Read the model definition and answer for the solid it produces. Units are mm, in the model's axes. A direction names the side the tool comes from. Give positions to 0.01 mm unless a question says otherwise; leave off trailing zeros. Order: outer loops, then holes, each group sorted by start corner. A loop starts at its lowest first (then second) coordinate and runs counter-clockwise, first axis right, second up.
```python
from build123d import *

# Parameters (mm, degrees)
SKETCH2_W           = 98
SKETCH2_H           = 62
BOSS_EXTRUDE1_DEPTH = 25
SKETCH3_W           = 9.5
SKETCH3_H           = 12
BOSS_EXTRUDE4_DEPTH = 1
SKETCH3_5_W         = 9.5
SKETCH3_5_H         = 12
CUT_EXTRUDE1_DEPTH  = 1
SKETCH4_R           = 3.25
CUT_EXTRUDE2_DEPTH  = 10
SKETCH5_R           = 0.5
BOSS_EXTRUDE5_DEPTH = 8
SKETCH6_W           = 7
SKETCH6_H           = 14
CUT_EXTRUDE9_DEPTH  = 10
SKETCH7_W           = 1.559437484
SKETCH7_H           = 10
BOSS_EXTRUDE6_DEPTH = 9
SKETCH8_W           = 15
SKETCH8_H           = 10
BOSS_EXTRUDE7_DEPTH = 2
BOSS_EXTRUDE7_TAPER = 30
FILLET5_R           = 2
SKETCH10_R          = 2.5
CUT_EXTRUDE10_DEPTH = 6
SKETCH11_R          = 0.5
CUT_EXTRUDE11_DEPTH = 3


with BuildPart() as part:
    # Sketch2 → Boss-Extrude1 (new body)
    with BuildSketch(Plane(origin=(0, 0, 0), x_dir=(1, 0, 0), z_dir=(0, 1, 0))):
        Rectangle(SKETCH2_W, SKETCH2_H)
    extrude(amount=BOSS_EXTRUDE1_DEPTH)

    # Sketch3 → Boss-Extrude4 (add)
    with BuildSketch(Plane.ZY.offset(49)):
        with Locations((-18.656971736, 15)):
            Rectangle(SKETCH3_W, SKETCH3_H)
    extrude(amount=-BOSS_EXTRUDE4_DEPTH)

    # Sketch3_5 → Cut-Extrude1 (cut)
    with BuildSketch(Plane.ZY.offset(49)):
        with Locations((-18.656971736, 15)):
            Rectangle(SKETCH3_5_W, SKETCH3_5_H)
    extrude(amount=-CUT_EXTRUDE1_DEPTH, mode=Mode.SUBTRACT)

    # Sketch4 → Cut-Extrude2 (cut)
    with BuildSketch(Plane.ZY.offset(48)):
        with Locations((-18.406971736, 16)):
            Circle(SKETCH4_R)
    extrude(amount=-CUT_EXTRUDE2_DEPTH, mode=Mode.SUBTRACT)

    # Sketch5 → Boss-Extrude5 (add)
    with BuildSketch(Plane.ZY.offset(38)):
        with Locations((-18.406971736, 16)):
            Circle(SKETCH5_R)
    extrude(amount=BOSS_EXTRUDE5_DEPTH)

    # Sketch6 → Cut-Extrude9 (cut)
    with BuildSketch(Plane.ZY.offset(49)):
        with Locations((-6.406971736, 14)):
            Rectangle(SKETCH6_W, SKETCH6_H)
    extrude(amount=-CUT_EXTRUDE9_DEPTH, mode=Mode.SUBTRACT)

    # Sketch7 → Boss-Extrude6 (add)
    with BuildSketch(Plane.ZY.offset(39)):
        with Locations((-4.686690478, 14)):
            Rectangle(SKETCH7_W, SKETCH7_H)
    extrude(amount=BOSS_EXTRUDE6_DEPTH)

    # Sketch8 → Boss-Extrude7 (add)
    with BuildSketch(Plane.ZY.offset(49)):
        with Locations((12.093028264, 15)):
            Rectangle(SKETCH8_W, SKETCH8_H)
    extrude(amount=BOSS_EXTRUDE7_DEPTH, taper=BOSS_EXTRUDE7_TAPER)

    # Fillet5
    fillet5_edges = [part.edges().sort_by_distance(p)[0] for p in [
        (0, 25, 31),
        (-49, 25, 0),
        (0, 25, -31),
        (-49, 0, 0),
        (0, 0, 31),
        (49, 0, 0),
        (0, 0, -31),
        (49, 25, 0),
        (-49, 12.5, -31),
        (-49, 12.5, 31),
        (49, 12.5, 31),
        (49, 12.5, -31),
    ]]
    fillet(fillet5_edges, radius=FILLET5_R)

    # Sketch10 → Cut-Extrude10 (cut)
    with BuildSketch(Plane.XZ):
        with Locations(Location((-43, -25.5, 0), (0, 0, 270))):
            Circle(SKETCH10_R)
        with Locations(Location((-43, 25.5, 0), (0, 0, 270))):
            Circle(SKETCH10_R)
        with Locations(Location((43, 25.5, 0), (0, 0, 270))):
            Circle(SKETCH10_R)
        with Locations(Location((43, -25.5, 0), (0, 0, 270))):
            Circle(SKETCH10_R)
    extrude(amount=-CUT_EXTRUDE10_DEPTH, mode=Mode.SUBTRACT)

    # Sketch11 → Cut-Extrude11 (cut)
    with BuildSketch(Plane(origin=(0, 25, 0), x_dir=(1, 0, 0), z_dir=(0, 1, 0))):
        with Locations(Location((-33, 16.5, 0), (0, 0, 270))):
            Circle(SKETCH11_R)
        with Locations(Location((-33, 10.5, 0), (0, 0, 270))):
            Circle(SKETCH11_R)
        with Locations(Location((-33, 4.5, 0), (0, 0, 270))):
            Circle(SKETCH11_R)
        with Locations(Location((-33, -1.5, 0), (0, 0, 270))):
            Circle(SKETCH11_R)
        with Locations(Location((-33, -7.5, 0), (0, 0, 270))):
            Circle(SKETCH11_R)
    extrude(amount=-CUT_EXTRUDE11_DEPTH, mode=Mode.SUBTRACT)


solid = part.part
```
1) Given pin 1 (5 mm diameter, centred on y = 6.5, z = 19.5, fed in from -X); pin 2 (0.8 mm diameter, centred on x = -33, z = -16.5, fed in from +Y); pin 3 (2.5 mm diameter, centred on x = -44, z = 26, fed in from -Y), each flat-ended and moving along its own axis, determine where each tip first touches the part or whether it passes through.
Final values:
pin 1: stops at x = -49
pin 2: stops at y = 22
pin 3: stops at y = 6
2) The part is cut by section C-C on z = -25.5. Determine the outline of the cut face in (x, y).
Final values:
outline: (-49, 2) arc R2 ccw to (-47, 0) - (-45.5, 0) - (-45.5, 6) - (-40.5, 6) - (-40.5, 0) - (40.5, 0) - (40.5, 6) - (45.5, 6) - (45.5, 0) - (47, 0) arc R2 ccw to (49, 2) - (49, 23) arc R2 ccw to (47, 25) - (-47, 25) arc R2 ccw to (-49, 23) - close
3) Consider L1, parallel to Z at x = -33, y = 22.9; L2, parallel to X at y = 4.15, z = 25.5; L3, parallel to Z at x = -33, y = 23.45. Determine where each line is inside the solid, lowest interval first.
Final values:
L1: z = -31 to -17, -16 to -11, -10 to -5, -4 to 1, 2 to 7, 8 to 31
L2: x = -49 to -45.5, -40.5 to 40.5, 45.5 to 49
L3: z = -30.95 to -17, -16 to -11, -10 to -5, -4 to 1, 2 to 7, 8 to 30.95
4) The part is cut by section B-B on y = 4.75. Determine the outline of the cut face in (x, z).
Final values:
outline: (-49, -29) arc R2 ccw to (-47, -31) - (47, -31) arc R2 ccw to (49, -29) - (49, 29) arc R2 ccw to (47, 31) - (-47, 31) arc R2 ccw to (-49, 29) - close; hole circle Ø5 at (-43, -25.5); hole circle Ø5 at (-43, 25.5); hole circle Ø5 at (43, -25.5); hole circle Ø5 at (43, 25.5)
5) For a pull along Z with two mould halves and no side action, classify faces 1 (the face through (-38, 15, -18)), 2 (the face through (-1, 12, -31)), 3 (the face through (-1, 12, 31)), 4 (the face through (-51, 15, 12)) as released by +Z, released by -Z, zero draft, split by the parting line, or undercut.
Final values:
face 1: undercut
face 2: released by -Z
face 3: released by +Z
face 4: zero draft
6) A tool of negligible diameter and unlimited length cuts with its end or side. For faces 5 (the face through (0.66, 24.4, 30.43)), 6 (the face through (-44, 7, -6)), 7 (the face through (43, 6, 26)), from which of +Z, -Z, +X, -X, +Y, -Y can it reach the whole face along a straight path? Write none if from no direction.
Final values:
face 5: +Z, +X, -X, +Y
face 6: -X
face 7: -Y
7) The part is cut by section A-A on x = -43. Determine the outline of the cut face in (y, z).
Final values:
outline: (0, -29) arc R2 ccw to (2, -31) - (23, -31) arc R2 ccw to (25, -29) - (25, 29) arc R2 ccw to (23, 31) - (2, 31) arc R2 ccw to (0, 29) - (0, 28) - (6, 28) - (6, 23) - (0, 23) - (0, -23) - (6, -23) - (6, -28) - (0, -28) - close; (9, -5.47) - (19, -5.47) - (19, -3.91) - (9, -3.91) - close; circle Ø1 at (16, -18.41); hole (7, -9.91) - (21, -9.91) - (21, -2.91) - (7, -2.91) - close; hole circle Ø6.5 at (16, -18.41)
